Source: CAD feature listing. Evaluate the final solid. Frame: model axes, mm. Coordinates: 2 decimals unless noted, no trailing zeros. Order: outer loops, then holes, each group sorted by start corner. A loop starts at its lowest first (then second) coordinate and runs counter-clockwise, first axis right, second up. Notation, with made-up numbers: (51.5, 63.5) -> (99.5, 63.5) arc R28 ccw to (99.5, 84.5) -> close; hole circle Ø5 at (49, 59). An arc over 180 degrees is marked (long way). Write item = value, one per line. Start each with the question number.
Item 1: Section query A-A (z = -51). Output: boundary loops of the cut face in (x, y), then the cut area to 3 significant figures.
Item 2: Ray query, line 1 along Z through (x, y) = (-5, -3); line 2 along Z through (x, y) = (-8.5, -1.5); line 3 along Y through (x, z) = (-5.5, 27). Return the intervals inside material, ascending. Write a range as [from, to].
Item 3: Contact query for flat-ended pins moving along their axis: pin 1 (4 mm diameter, centred on y = -28.85, z = 93.88, fed in from -X); pin 2 (6 mm diameter, centred on y = 40.31, z = -10.69, fed in from -X). Output: stop coordinate, or through.
Item 4: Section query B-B (x = -7.5). Count the separate pieces of the cut face and the enclosed holes in it, then the cut area to 3 significant figures.
Item 5: Section query C-C (z = -86). Output: boundary loops of the cut face in (x, y), then the cut area to 3 significant figures.
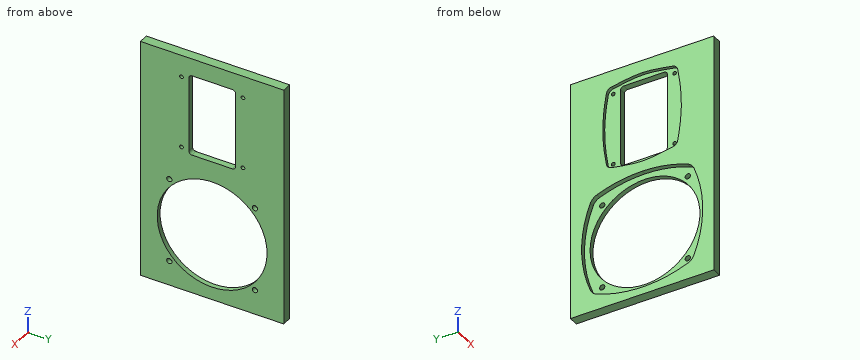
```python
from build123d import *

# Parameters (mm, degrees)
F1_DEPTH = 9
F0_R     = 2.5
F0_R_2   = 51.75
F2_DEPTH = 4.5
F0_R_3   = 3
F0_R_4   = 1.75
F3_R     = 11
F4_DEPTH = 6
F5_R     = 6


# Not quite as in the source:
# - a feature names something its author has since deleted; it is built from what else it names


with BuildPart() as f1:
    # F0 (on Right) → F1 (new body)
    with BuildSketch(Plane.YZ):
        Polygon((67.5, -115), (67.5, 115), (0, 115), (-67.5, 115), (-67.5, -115), align=None)
        with BuildLine():
            ThreePointArc((-47.0226009489, -3.9773990511), (-24.0347326375, 3.4781900517), (0, 6))
            ThreePointArc((0, 6), (24.0347326375, 3.4781900517), (47.0226009489, -3.9773990511))
            ThreePointArc((47.0226009489, -3.9773990511), (57, -51), (47.0226009489, -98.0226009489))
            ThreePointArc((47.0226009489, -98.0226009489), (0, -108), (-47.0226009489, -98.0226009489))
            ThreePointArc((-47.0226009489, -98.0226009489), (-57, -51), (-47.0226009489, -3.9773990511))
        make_face(mode=Mode.SUBTRACT)
        with BuildLine():
            add(Edge.make_bspline(
                [(0, 102.9074018363), (-10.9007532398, 102.8937314348), (-21.8015064796, 100.0876465048), (-32.7022597194, 98.4757185701)],
                knots=[0.5012187781, 0.5012187781, 0.5012187781, 0.5012187781, 1, 1, 1, 1], degree=3))
            add(Edge.make_bspline(
                [(32.8620764687, 98.4757185701), (21.934687104, 100.0915852706), (10.9806616144, 102.9143158042), (0.0266361249, 102.9074352401), (0, 102.9074018363)],
                knots=[0, 0, 0, 0, 0.5, 0.5012187781, 0.5012187781, 0.5012187781, 0.5012187781], degree=3))
            add(Edge.make_bspline(
                [(32.8620764687, 20.339185372), (35.4709924216, 33.361940905), (38.6888243276, 59.4074519711), (35.4709924216, 85.4529630371), (32.8620764687, 98.4757185701)],
                knots=[0, 0, 0, 0, 0.5, 1, 1, 1, 1], degree=3))
            add(Edge.make_bspline(
                [(0, 15.9075021058), (0.0266361249, 15.907468702), (10.9806616144, 15.9005881379), (21.934687104, 18.7233186715), (32.8620764687, 20.339185372)],
                knots=[0.4987812219, 0.4987812219, 0.4987812219, 0.4987812219, 0.5, 1, 1, 1, 1], degree=3))
            add(Edge.make_bspline(
                [(-32.7022597194, 20.339185372), (-21.8015064796, 18.7272574373), (-10.9007532398, 15.9211725073), (0, 15.9075021058)],
                knots=[0, 0, 0, 0, 0.4987812219, 0.4987812219, 0.4987812219, 0.4987812219], degree=3))
            add(Edge.make_bspline(
                [(-32.7022597194, 98.4757185701), (-35.3111756724, 85.4529630371), (-38.5290075784, 59.4074519711), (-35.3111756724, 33.361940905), (-32.7022597194, 20.339185372)],
                knots=[0, 0, 0, 0, 0.5, 1, 1, 1, 1], degree=3))
        make_face(mode=Mode.SUBTRACT)
    extrude(amount=-F1_DEPTH)

    # F0 (on Right) → F2 (join)
    with BuildSketch(Plane.YZ):
        with BuildLine():
            ThreePointArc((47.0226009489, -3.9773990511), (24.0347326375, 3.4781900517), (0, 6))
            ThreePointArc((0, 6), (-24.0347326375, 3.4781900517), (-47.0226009489, -3.9773990511))
            ThreePointArc((-47.0226009489, -3.9773990511), (-57, -51), (-47.0226009489, -98.0226009489))
            ThreePointArc((-47.0226009489, -98.0226009489), (0, -108), (47.0226009489, -98.0226009489))
            ThreePointArc((47.0226009489, -98.0226009489), (57, -51), (47.0226009489, -3.9773990511))
        make_face()
        with Locations((-40.3050865276, -91.3050865276)):
            Circle(F0_R, mode=Mode.SUBTRACT)
        with Locations((-40.3050865276, -10.6949134724)):
            Circle(F0_R, mode=Mode.SUBTRACT)
        with Locations((40.3050865276, -91.3050865276)):
            Circle(F0_R, mode=Mode.SUBTRACT)
        with Locations((0, -51)):
            Circle(F0_R_2, mode=Mode.SUBTRACT)
        with Locations((40.3050865276, -10.6949134724)):
            Circle(F0_R, mode=Mode.SUBTRACT)
    extrude(amount=-F2_DEPTH)

    # F3
    f3_edges = [f1.edges().sort_by_distance(p)[0] for p in [
        (-6.75, 47.022601, -3.977399),
        (-6.75, -47.022601, -3.977399),
        (-6.75, -47.022601, -98.022601),
        (-6.75, 47.022601, -98.022601),
    ]]
    fillet(f3_edges, radius=F3_R)



with BuildPart() as f2:
    # F0 (on Right) → F2, piece 2 (new body)
    with BuildSketch(Plane.YZ):
        with Locations((-28.8455340613, 24.9354520307)):
            Circle(F0_R_3)
        with Locations((-28.8455340613, 24.9354520307)):
            Circle(F0_R_4, mode=Mode.SUBTRACT)
    extrude(amount=-F2_DEPTH)


with BuildPart() as f2b:
    # F0 (on Right) → F2, piece 3 (new body)
    with BuildSketch(Plane.YZ):
        with Locations((29.0053508105, 24.9354520307)):
            Circle(F0_R_3)
        with Locations((29.0053508105, 24.9354520307)):
            Circle(F0_R_4, mode=Mode.SUBTRACT)
    extrude(amount=-F2_DEPTH)


with BuildPart() as f1_1:
    add(f1.part)

    add(f2.part)  # F4 merges F2

    add(f2b.part)  # F4 merges F2b
    # F0 (on Right) → F4 (join)
    with BuildSketch(Plane.YZ):
        with BuildLine():
            add(Edge.make_bspline(
                [(32.8620764687, 98.4757185701), (21.934687104, 100.0915852706), (10.9806616144, 102.9143158042), (0.0266361249, 102.9074352401), (0, 102.9074018363)],
                knots=[0, 0, 0, 0, 0.5, 0.5012187781, 0.5012187781, 0.5012187781, 0.5012187781], degree=3))
            Line((0, 102.9074018363), (0, 98.4074519711))
            Line((0, 98.4074519711), (19.0799083746, 98.4074519711))
            ThreePointArc((19.0799083746, 98.4074519711), (21.2012287182, 97.5287723146), (22.0799083746, 95.4074519711))
            Line((22.0799083746, 95.4074519711), (22.0799083746, 23.4074519711))
            ThreePointArc((22.0799083746, 23.4074519711), (21.2012287182, 21.2861316275), (19.0799083746, 20.4074519711))
            Line((19.0799083746, 20.4074519711), (0, 20.4074519711))
            Line((0, 20.4074519711), (0, 15.9075021058))
            add(Edge.make_bspline(
                [(0, 15.9075021058), (0.0266361249, 15.907468702), (10.9806616144, 15.9005881379), (21.934687104, 18.7233186715), (32.8620764687, 20.339185372)],
                knots=[0.4987812219, 0.4987812219, 0.4987812219, 0.4987812219, 0.5, 1, 1, 1, 1], degree=3))
            add(Edge.make_bspline(
                [(32.8620764687, 20.339185372), (35.4709924216, 33.361940905), (38.6888243276, 59.4074519711), (35.4709924216, 85.4529630371), (32.8620764687, 98.4757185701)],
                knots=[0, 0, 0, 0, 0.5, 1, 1, 1, 1], degree=3))
        make_face()
        with Locations((29.0053508105, 24.9354520307)):
            Circle(F0_R_3, mode=Mode.SUBTRACT)
        with Locations((29.0053508105, 93.8794519114)):
            Circle(F0_R_3, mode=Mode.SUBTRACT)
        with BuildLine():
            Line((0, 98.4074519711), (0, 102.9074018363))
            add(Edge.make_bspline(
                [(0, 102.9074018363), (-10.9007532398, 102.8937314348), (-21.8015064796, 100.0876465048), (-32.7022597194, 98.4757185701)],
                knots=[0.5012187781, 0.5012187781, 0.5012187781, 0.5012187781, 1, 1, 1, 1], degree=3))
            add(Edge.make_bspline(
                [(-32.7022597194, 98.4757185701), (-35.3111756724, 85.4529630371), (-38.5290075784, 59.4074519711), (-35.3111756724, 33.361940905), (-32.7022597194, 20.339185372)],
                knots=[0, 0, 0, 0, 0.5, 1, 1, 1, 1], degree=3))
            add(Edge.make_bspline(
                [(-32.7022597194, 20.339185372), (-21.8015064796, 18.7272574373), (-10.9007532398, 15.9211725073), (0, 15.9075021058)],
                knots=[0, 0, 0, 0, 0.4987812219, 0.4987812219, 0.4987812219, 0.4987812219], degree=3))
            Line((0, 15.9075021058), (0, 20.4074519711))
            Line((0, 20.4074519711), (-18.9200916254, 20.4074519711))
            ThreePointArc((-18.9200916254, 20.4074519711), (-21.0414119689, 21.2861316275), (-21.9200916254, 23.4074519711))
            Line((-21.9200916254, 23.4074519711), (-21.9200916254, 95.4074519711))
            ThreePointArc((-21.9200916254, 95.4074519711), (-21.0414119689, 97.5287723146), (-18.9200916254, 98.4074519711))
            Line((-18.9200916254, 98.4074519711), (0, 98.4074519711))
        make_face()
        with Locations((-28.8455340613, 24.9354520307)):
            Circle(F0_R_3, mode=Mode.SUBTRACT)
        with Locations((-28.8455340613, 93.8794519114)):
            Circle(F0_R_3, mode=Mode.SUBTRACT)
        with Locations((29.0053508105, 93.8794519114)):
            Circle(F0_R_3)
        with Locations((29.0053508105, 93.8794519114)):
            Circle(F0_R_4, mode=Mode.SUBTRACT)
        with Locations((-28.8455340613, 93.8794519114)):
            Circle(F0_R_3)
        with Locations((-28.8455340613, 93.8794519114)):
            Circle(F0_R_4, mode=Mode.SUBTRACT)
        with Locations((-28.8455340613, 24.9354520307)):
            Circle(F0_R_3)
        with Locations((-28.8455340613, 24.9354520307)):
            Circle(F0_R_4, mode=Mode.SUBTRACT)
        with Locations((29.0053508105, 24.9354520307)):
            Circle(F0_R_3)
        with Locations((29.0053508105, 24.9354520307)):
            Circle(F0_R_4, mode=Mode.SUBTRACT)
    extrude(amount=-F4_DEPTH)

    # F5
    f5_edges = [f1_1.edges().sort_by_distance(p)[0] for p in [
        (-7.5, 32.862076, 98.475719),
        (-7.5, 32.862076, 20.339185),
        (-7.5, -32.70226, 20.339185),
        (-7.5, -32.70226, 98.475719),
    ]]
    fillet(f5_edges, radius=F5_R)


solid = f1_1.part
```
Computed:
q1.outline = (-9, -67.5) -> (0, -67.5) -> (0, -51.75) -> (-4.5, -51.75) -> (-4.5, -57) -> (-9, -57) -> close; (-9, 57) -> (-4.5, 57) -> (-4.5, 51.75) -> (0, 51.75) -> (0, 67.5) -> (-9, 67.5) -> close
q1.area = 236 mm^2
q2.line_1 = [-115, -107.96], [5.96, 20.41], [98.41, 115]
q2.line_2 = [-115, -107.99], [5.99, 15.93], [102.89, 115]
q2.line_3 = [-67.5, -21.92], [22.08, 67.5]
q3.pin_1 = -6
q3.pin_2 = -4.5
q4.separate_pieces = 1
q4.enclosed_holes = 2
q4.area = 13,800 mm^2
q5.outline = (-9, -67.5) -> (0, -67.5) -> (0, -38.12) -> (-4.5, -38.12) -> (-4.5, -51.58) -> (-9, -51.58) -> close; (-9, 51.58) -> (-4.5, 51.58) -> (-4.5, 38.12) -> (0, 38.12) -> (0, 67.5) -> (-9, 67.5) -> close
q5.area = 408 mm^2
